```python
from build123d import *

# Parameters (mm, degrees)
F0_R     = 13.55
F1_DEPTH = 7


with BuildPart() as f1:
    # F0 (on Top) → F1 (new body)
    with BuildSketch(Plane.XY):
        with BuildLine():
            ThreePointArc((-19.002935, 19.291424), (-14.526693, 6.593441), (-27.753296, 4.076997))
            Line((-27.753296, 4.076997), (-70.395388, -42.391945))
            Line((-70.395388, -42.391945), (-9.481418, -28.723067))
            ThreePointArc((-9.481418, -28.723067), (-7.062366, -21.723421), (0, -19.494107))
            ThreePointArc((0, -19.494107), (7.062366, -21.723421), (9.481418, -28.723067))
            Line((9.481418, -28.723067), (70.395388, -42.391945))
            Line((70.395388, -42.391945), (27.753296, 4.076997))
            ThreePointArc((27.753296, 4.076997), (14.526693, 6.593441), (19.002935, 19.291424))
            Line((19.002935, 19.291424), (0, 74.57269))
            Line((0, 74.57269), (-19.002935, 19.291424))
        make_face()
        with Locations((-28.363841, -17.090467)):
            Circle(F0_R, mode=Mode.SUBTRACT)
        with Locations((28.22023, -17.173382)):
            Circle(F0_R, mode=Mode.SUBTRACT)
        Circle(F0_R, mode=Mode.SUBTRACT)
        with Locations((0, 31.871319)):
            Circle(F0_R, mode=Mode.SUBTRACT)
    extrude(amount=F1_DEPTH)


solid = f1.part
```
The model under review builds one solid part; all positions refer to its coordinate system, in mm. A direction names the side the tool comes from. Round coordinates to 2 decimals unless told otherwise and drop trailing zeros. Loops run counter-clockwise (first coordinate to the right, second up) from the corner with the lowest first, then second, coordinate; pieces in that order, holes last. Notation, with made-up numbers: (83.5, 84) -> (87.5, 84) arc R30 cw to (87.5, 117) -> close; hole circle Ø1 at (42.25, 76). An arc over 180 degrees is marked (long way). Answer in a Markdown table with one row per item.
1) Consider section D-D, the plane z = 2. Write out the cut boundary in (x, y), plus the area to 3 significant figures.
Taken from the geometry:
| item | result |
|---|---|
| outline | (-70.4, -42.39) -> (-9.48, -28.72) arc R8.24 cw to (0, -19.49) arc R8.24 cw to (9.48, -28.72) -> (70.4, -42.39) -> (27.75, 4.08) arc R8.88 cw (long way) to (19, 19.29) -> (0, 74.57) -> (-19, 19.29) arc R8.88 cw (long way) to (-27.75, 4.08) -> close; hole circle Ø27.1 at (-28.36, -17.09); hole circle Ø27.1 at (0, 0); hole circle Ø27.1 at (0, 31.87); hole circle Ø27.1 at (28.22, -17.17) |
| area | 2,480 mm² |
2) Draft analysis for pull direction X (two halves, no side actions). For faces 1 (the flat face through (-48.776, -18.832, 3.451)), 2 (the cylindrical face through (6.985, -21.649, 3.451)), 3 (the flat face through (49.37, -19.48, 3.45)), 4 (the flat face through (0, -14, 7)), state which applies: pulls with the +X half, pulls with the -X half, needs draft (parallel to the pull), parting line crosses it, or undercut.
Taken from the geometry:
| item | result |
|---|---|
| face 1 | pulls with the -X half |
| face 2 | undercut |
| face 3 | pulls with the +X half |
| face 4 | needs draft |
3) Tool access review of faces 5 (the flat face through (-40.365, -35.653, 3.451)), 6 (the cylindrical face through (-2.937, 18.644, 3.451)): name each direction out of +Z, -Z, +X, -X, +Y, -Y from which nothing blocks a thin tool from reaching the whole face with its end or side.
Taken from the geometry:
| item | result |
|---|---|
| face 5 | +Z, -Z, -Y |
| face 6 | +Z, -Z |
4) Consider section A-A, the plane y = 0. Write out the cut boundary in (x, z), plus the area to 3 significant figures.
Taken from the geometry:
| item | result |
|---|---|
| outline | (-31.49, 0) -> (-13.55, 0) -> (-13.55, 7) -> (-31.49, 7) -> close; (13.55, 0) -> (31.49, 0) -> (31.49, 7) -> (13.55, 7) -> close |
| area | 251 mm² |
5) Consider section B-B, the plane x = -39. Write out the cut boundary in (y, z).
Taken from the geometry:
| item | result |
|---|---|
| outline | (-35.35, 0) -> (-25.49, 0) -> (-25.49, 7) -> (-35.35, 7) -> close; (-8.7, 0) -> (-8.18, 0) -> (-8.18, 7) -> (-8.7, 7) -> close |
6) Consider section C-C, the plane y = -25. Write out the cut boundary in (x, z).
Taken from the geometry:
| item | result |
|---|---|
| outline | (-54.44, 0) -> (-39.37, 0) -> (-39.37, 7) -> (-54.44, 7) -> close; (-17.36, 0) -> (-9.12, 0) -> (-9.12, 7) -> (-17.36, 7) -> close; (9.12, 0) -> (17.16, 0) -> (17.16, 7) -> (9.12, 7) -> close; (39.28, 0) -> (54.44, 0) -> (54.44, 7) -> (39.28, 7) -> close |
7) Wall thickness on line 1 along X through (y, z) = (-12.5, 0.5); line 2 along X through (y, z) = (-6, 2.25); line 3 along X through (y, z) = (32, 2.5): over which ranges is each line inside the solid? List them lowest first.
Taken from the geometry:
| item | result |
|---|---|
| line 1 | x = -42.97 to -41.11, -15.62 to -5.23, 5.23 to 15.5, 40.94 to 42.97 |
| line 2 | x = -37 to -36.15, -20.58 to -12.15, 12.15 to 20.55, 35.89 to 37 |
| line 3 | x = -14.63 to -13.55, 13.55 to 14.63 |
8) For pin 1 Ø3 at (y, z) = (45, 4.5) entering from +X; pin 2 Ø2 at (y, z) = (54, 6) entering from -X; pin 3 Ø2 at (x, z) = (-36, 3) entering from -Y, all flat-tipped, find the tip position at first contact; note any pin that passes through.
Taken from the geometry:
| item | result |
|---|---|
| pin 1 | stops at x = 10.68 |
| pin 2 | stops at x = -7.42 |
| pin 3 | stops at y = -34.9 |
